from build123d import *

# Parameters (mm, degrees)
F0_R     = 18.5
F1_DEPTH = 1.7
F2_R     = 17
F3_DEPTH = 2
F4_SIZE  = 0.5
F5_R     = 1
F6_W     = 20
F6_H     = 55.344078
F7_DEPTH = 1.7


with BuildPart() as f1:
    # F0 (on Top) → F1 (new body)
    with BuildSketch(Plane.XY):
        Circle(F0_R)
    extrude(amount=F1_DEPTH)

    # F2 (on face) → F3 (join)
    with BuildSketch(Plane.XY.offset(1.7)):
        Circle(F2_R)
    extrude(amount=F3_DEPTH)

    # F4
    f4_edges = [f1.edges().sort_by_distance(p)[0] for p in [
        (-17, 0, 3.7),
    ]]
    chamfer(f4_edges, length=F4_SIZE)

    # F5
    f5_edges = [f1.edges().sort_by_distance(p)[0] for p in [
        (-18.5, 0, 0),
    ]]
    fillet(f5_edges, radius=F5_R)

    # F6 (on face) → F7 (cut)
    with BuildSketch(Plane(origin=(0, 0, 0), x_dir=(1, 0, 0), z_dir=(0, 0, -1))):
        Rectangle(F6_W, F6_H)
    extrude(amount=-F7_DEPTH, mode=Mode.SUBTRACT)


solid = f1.part
Can you work these out from the model? Positions are in its coordinate system, mm. A direction names the side the tool comes from. Give positions to 0.01 mm unless a question says otherwise; leave off trailing zeros. Loops run counter-clockwise (first coordinate to the right, second up) from the corner with the lowest first, then second, coordinate; pieces in that order, holes last. Notation, with made-up numbers: (-11, -28.5) - (0, -28.5) arc R16 cw to (0, -23.5) - close; hole circle Ø3 at (-26, -34). An arc over 180 degrees is marked (long way). Answer as a JSON object with one key per item and string values.
Q1. Imagine slicing it at C-C on z = 2.7. Write out the boundary of the cut face in (x, y).
Geometry says:
{"outline": "circle Ø34 at (0, 0)"}
Q2. Will these pins go through, and if not, where does the flat tip stop? P1, Ø0.5, axis at y = 6, z = 1.5, coming from the +X side; P2, Ø6, axis at x = 3.5, y = 4, coming from the -Z side; P3, Ø12, axis at x = 12.5, y = -4, coming from the -Z side; P4, Ø0.9, axis at y = 7, z = 0.5, coming from the -X side.
Geometry says:
{"P1": "x = 17.58", "P2": "z = 1.7", "P3": "z = 0", "P4": "x = -17.24"}
Q3. If we mould it in two halves opening along X, with no side actions, what happens to faces 4 (the flat face through (0, 0, 1.7)), 5 (the flat face through (-17.4, 0.1, 1.7)), 6 (the cylindrical face through (-18.5, 0.26, 1.35))? For each: pulls with the +X half, pulls with the -X half, needs draft (parallel to the pull), parting line crosses it, or undercut.
Geometry says:
{"face 4": "undercut", "face 5": "needs draft", "face 6": "pulls with the -X half"}
Q4. Imagine slicing it at D-D on y = -15. Give the number of separate pieces and of enclosed holes in the cut face, plus the area to 3 significant figures.
Geometry says:
{"separate pieces": "3", "enclosed holes": "0", "area": "33.6 mm²"}
Q5. Which directions (+Z, -Z, +X, -X, +Y, -Y) give clear straight access to the entire face, cutting with the end or side of a thin tool? Please do faces 1 (the cylindrical face through (9.139, 14.334, 2.44)), 2 (the flat face through (17.4, 0.1, 1.7)), 3 (the flat face through (10, 0, 1)).
Geometry says:
{"face 1": "+Z", "face 2": "+Z, +X", "face 3": "-Z, +Y, -Y"}
Q6. Imagine slicing it at B-B on x = 0. Write out the boundary of the cut face in (y, z), plus the area to 4 significant figures.
Geometry says:
{"outline": "(-17, 1.7) - (17, 1.7) - (17, 3.2) - (16.5, 3.7) - (-16.5, 3.7) - (-17, 3.2) - close", "area": "67.75 mm²"}
Q7. If I drill on L1, parallel to Z at x = 6.5, y = -11; L2, parallel to X at y = -12.5, z = 1; L3, parallel to X at y = -9, z = 0.5, over which ranges is the centre line in solid material (lowest first)?
Geometry says:
{"L1": "1.7 to 3.7", "L2": "-13.64 to -10, 10 to 13.64", "L3": "-16.01 to -10, 10 to 16.01"}
Q8. Imagine slicing it at A-A on y = 0. Write out the boundary of the cut face in (x, z).
Geometry says:
{"outline": "(-18.5, 1) arc R1 ccw to (-17.5, 0) - (-10, 0) - (-10, 1.7) - (10, 1.7) - (10, 0) - (17.5, 0) arc R1 ccw to (18.5, 1) - (18.5, 1.7) - (17, 1.7) - (17, 3.2) - (16.5, 3.7) - (-16.5, 3.7) - (-17, 3.2) - (-17, 1.7) - (-18.5, 1.7) - close"}
